```python
from build123d import *

# Parameters (mm, degrees)
F0_W      = 50
F0_H      = 26
F1_DEPTH  = 55
F3_DEPTH  = 45
F4_R      = 2
F5_R      = 2
F6_W      = 55
F6_H      = 31
F7_DEPTH  = 120
F9_DEPTH  = 110
F10_R     = 2
F11_W     = 193.8701719046
F11_H     = 235.1342812181
F12_DEPTH = 15.501
F13_R     = 3.5
F14_DEPTH = 3
F14_TAPER = 3
F15_R     = 3.5
F16_DEPTH = 3
F16_TAPER = 3
F18_DEPTH = 55


with BuildPart() as f1:
    # F0 (on Top) → F1 (new body)
    with BuildSketch(Plane.XY):
        Rectangle(F0_W, F0_H)
    extrude(amount=F1_DEPTH)

    # F2 (on face) → F3 (cut)
    with BuildSketch(Plane(origin=(0, 0, 0), x_dir=(1, 0, 0), z_dir=(0, 0, -1))):
        Polygon((-17.3603594806, -8), (17.3603594806, -8), (17.5, 0), (17.3603594806, 8), (-17.3603594806, 8), (-17.5, 0), align=None)
    extrude(amount=-F3_DEPTH, mode=Mode.SUBTRACT)

    # F4
    f4_edges = [f1.edges().sort_by_distance(p)[0] for p in [
        (-17.360359, 8, 22.5),
        (17.360359, 8, 22.5),
    ]]
    fillet(f4_edges, radius=F4_R)

    # F5
    f5_edges = [f1.edges().sort_by_distance(p)[0] for p in [
        (-17.360359, -8, 22.5),
        (17.360359, -8, 22.5),
    ]]
    fillet(f5_edges, radius=F5_R)

    # F6 (on face) → F7 (join)
    with BuildSketch(Plane(origin=(0, 0, 0), x_dir=(1, 0, 0), z_dir=(0, 0, -1))):
        Rectangle(F6_W, F6_H)
    extrude(amount=F7_DEPTH)

    # F8 (on face) → F9 (cut)
    with BuildSketch(Plane.XY):
        Polygon((-19.8167218183, 10.5), (-20, 0), (-19.8167218183, -10.5), (19.8167218183, -10.5), (20, 0), (19.8167218183, 10.5), align=None)
    extrude(amount=-F9_DEPTH, mode=Mode.SUBTRACT)

    # F10
    f10_edges = [f1.edges().sort_by_distance(p)[0] for p in [
        (-19.816722, -10.5, -55),
        (19.816722, -10.5, -55),
        (-19.816722, 10.5, -55),
        (19.816722, 10.5, -55),
    ]]
    fillet(f10_edges, radius=F10_R)

    # F11 (on Front) → F12 (cut, through all)
    with BuildSketch(Plane.XZ):
        with Locations((2.0464733243, -30.8961831033)):
            Rectangle(F11_W, F11_H)
    extrude(amount=-F12_DEPTH, mode=Mode.SUBTRACT)

    # F13 (on face) → F14 (join)
    with BuildSketch(Plane(origin=(0, 0, 0), x_dir=(-1, 0, 0), z_dir=(0, 1, 0))):
        with Locations((0, 49.4391918182)):
            Circle(F13_R)
    extrude(amount=F14_DEPTH, taper=F14_TAPER)

    # F15 (on face) → F16 (join)
    with BuildSketch(Plane(origin=(0, 0, 0), x_dir=(-1, 0, 0), z_dir=(0, 1, 0))):
        with Locations((0, -114.7729158401)):
            Circle(F15_R)
    extrude(amount=F16_DEPTH, taper=F16_TAPER)

    # F17 (on face) → F18 (join, through all)
    with BuildSketch(Plane.XY):
        Polygon((-25, 0), (-27.5, 0), (-27.5, -15.5), (27.5, -15.5), (27.5, 0), (25, 0), (25, -13), (-25, -13), align=None)
    extrude(amount=F18_DEPTH)


solid = f1.part
```
Work out the finished part from the listing and answer in its coordinate system (mm). A direction names the side the tool comes from. Round coordinates to 2 decimals unless told otherwise and drop trailing zeros. Loops run counter-clockwise (first coordinate to the right, second up) from the corner with the lowest first, then second, coordinate; pieces in that order, holes last. Notation, with made-up numbers: (9.5, -29.5) -> (47.5, -29.5) arc R11 cw to (47.5, -14.5) -> close; hole circle Ø10 at (59, 36.5). An arc over 180 degrees is marked (long way). Write each question's results on one line, items separated by ' | '. Start each with the question number.
1. Section D-D (x = 0) is taken. Determine the outline of the cut face in (y, z), plus the area to 3 significant figures.
2. Section B-B (x = 9) is taken. Determine the outline of the cut face in (y, z), plus the area to 3 significant figures.
3. Given pin 1 Ø1.5 at (x, z) = (-3.5, -54) entering from +Y; pin 2 Ø1.5 at (x, z) = (-7, 26) entering from +Y, each flat-ended and moving along its own axis, determine where each tip first touches the part or whether it passes through.
4. Find the intervals of material crossed by probe 1 along Z at (x, y) = (-9, -0.5); probe 2 along X at (y, z) = (-1.5, 20); probe 3 along Y at (x, z) = (-21.5, -77), in increasing order. Write a range as from..to.
5. Section C-C (y = -3.75) is taken. Determine the outline of the cut face in (x, z), plus the area to 3 significant figures.
6. A tool of negligible diameter and unlimited length cuts with its end or side. For faces 5 (the face through (-27.5, -8, -34)), 6 (the face through (0, -4, 45)), from which of +Z, -Z, +X, -X, +Y, -Y can it reach the whole face along a straight path? Write none if from no direction.
7. For a pull along Z with two mould halves and no side action, classify faces 1 (the face through (0, -8, 55)), 2 (the face through (0.7, 1.9, -118.1)), 3 (the face through (0, 3, 49)), 4 (the face through (0, -8, 22)) as +Z half, -Z half, draft (parallel to the pull), parting line (faces both ways), or undercut.
8. Section A-A (z = -12) is taken. Determine the outline of the cut face in (x, y), plus the area to 3 significant figures.
Evaluation:
1) outline: (-15.5, -120) -> (0, -120) -> (0, -118.27) -> (3, -118.12) -> (3, -111.43) -> (0, -111.27) -> (0, -110) -> (-10.5, -110) -> (-10.5, 0) -> (-8, 0) -> (-8, 45) -> (0, 45) -> (0, 45.94) -> (3, 46.1) -> (3, 52.78) -> (0, 52.94) -> (0, 55) -> (-15.5, 55) -> close | area: 1,240 mm2
2) outline: (-15.5, -120) -> (0, -120) -> (0, -110) -> (-10.5, -110) -> (-10.5, 0) -> (-8, 0) -> (-8, 45) -> (0, 45) -> (0, 55) -> (-15.5, 55) -> close | area: 1,200 mm2
3) pin 1: stops at y = -10.5 | pin 2: stops at y = -8
4) probe 1: z = -120..-110, 45..55 | probe 2: x = -27.5..-17.47, 17.47..27.5 | probe 3: y = -15.5..0
5) outline: (-27.5, -120) -> (27.5, -120) -> (27.5, 55) -> (-27.5, 55) -> close; hole (-19.93, -110) -> (19.93, -110) -> (19.93, 0) -> (17.43, 0) -> (17.43, 45) -> (-17.43, 45) -> (-17.43, 0) -> (-19.93, 0) -> close | area: 3,670 mm2
6) face 5: +Z, -Z, -X, +Y, -Y | face 6: +Y
7) face 1: +Z half | face 2: undercut | face 3: draft | face 4: undercut
8) outline: (-27.5, -15.5) -> (27.5, -15.5) -> (27.5, 0) -> (20, 0) -> (19.85, -8.53) arc R2 cw to (17.85, -10.5) -> (-17.85, -10.5) arc R2 cw to (-19.85, -8.53) -> (-20, 0) -> (-27.5, 0) -> close | area: 436 mm2
